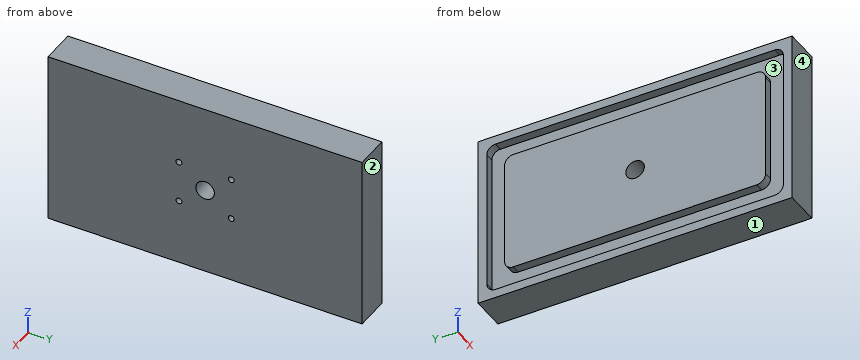
Autodesk Inventor part; units mm, degrees
ref_plane "YZ Plane" through (0, 0, 0) normal (1, 0, 0) x (0, 1, 0)
ref_plane "XZ Plane" through (0, 0, 0) normal (0, 1, 0) x (-1, 0, 0)
ref_plane "XY Plane" through (0, 0, 0) normal (0, 0, 1) x (1, 0, 0)
sketch "Sketch1" plane through (0, 0, 0) normal (1, 0, 0) x (0, 1, 0)
  line L0 (57.15, 31.75) -> (-57.15, 31.75)
  line L1 (-57.15, 31.75) -> (-57.15, -31.75)
  line L2 (-57.15, -31.75) -> (57.15, -31.75)
  line L3 (57.15, -31.75) -> (57.15, 31.75)
  line L4 (-50.8, 25.4) -> (50.8, 25.4)
  line L5 (50.8, 25.4) -> (50.8, -25.4)
  line L6 (50.8, -25.4) -> (-50.8, -25.4)
  line L7 (-50.8, -25.4) -> (-50.8, 25.4)
  point P0 (0, 0)
  point P1 (0, -31.75)
  point P2 (57.15, 0)
  point P3 (0, 25.4)
  point P4 (-50.8, 0)
  dimension "d0" = 63.5
  dimension "d1" = 114.3
  dimension "d14" = 50.8
  dimension "d15" = 101.6
extrude "Extrusion1" add sketch "Sketch1" along normal blind 12.7 contours L3 L2 L1 L0 | L4 L5 L6 L7
sketch "Sketch2" plane through (12.7, 0, 0) normal (1, 0, 0) x (0, 0, -1)
  line L0 (-7.62, -9.525) -> (7.62, 9.525) construction
  line L1 (-7.62, 9.525) -> (7.62, -9.525) construction
  circle A0 centre (0, 0) radius 3.3734
  dimension "d5" = 19.05
  dimension "d12" = 6.7469
  dimension "d13" = 15.24
sketch "Sketch3" plane through (0, 0, 0) normal (-1, 0, 0) x (0, 0, 1)
  line L0 (-28.575, -53.975) -> (28.575, -53.975)
  line L1 (28.575, -53.975) -> (28.575, 53.975)
  line L2 (28.575, 53.975) -> (-28.575, 53.975)
  line L3 (-28.575, 53.975) -> (-28.575, -53.975)
  line L4 (22.098, 47.498) -> (22.098, -47.498)
  line L5 (22.098, -47.498) -> (-22.098, -47.498)
  line L6 (-22.098, -47.498) -> (-22.098, 47.498)
  line L7 (-22.098, 47.498) -> (22.098, 47.498)
  point P0 (0, 0)
  point P1 (0, -53.975)
  point P2 (-28.575, 0)
  point P3 (0, 0)
  point P4 (28.575, 0)
  point P5 (0, 53.975)
  dimension "d16" = 107.95
  dimension "d17" = 57.15
  dimension "d31" = 6.477
extrude "Extrusion3" cut sketch "Sketch3" against normal blind 3.175
extrude "Extrusion4" cut sketch "Sketch2" against normal through all
hole "Hole1" at (12.7, -9.525, 7.62) at (12.7, 9.525, 7.62) at (12.7, 9.525, -7.62) at (12.7, -9.525, -7.62) direction (-1, 0, 0) diameter 2.159 depth 8.8646 tip angle 118
fillet "Fillet1" radius 3.175 8 edges at (1.5875, 53.975, 28.575) (1.5875, -47.498, 22.098) (1.5875, -47.498, -22.098) (1.5875, -53.975, -28.575) (1.5875, 47.498, -22.098) (1.5875, -53.975, 28.575) (1.5875, 53.975, -28.575) (1.5875, 47.498, 22.098)
properties part number "plate" material "Aluminum 6061"
Read the model definition and answer for the solid it produces. Units are mm, in the model's axes. Face numbers are marked on the shaded views. Give positions to 0.01 mm unless a question says otherwise; leave off trailing zeros. Write each loop counter-clockwise with the first axis right and the second up, starting at its lowest first coordinate (ties: lowest second). Pieces come first, ordered by that corner, then holes. Notation, with made-up numbers: (87.25, 14) -> (134.25, 14) arc R21 ccw to (134.25, 18) -> close; hole circle Ø11 at (43, 61.5). An arc over 180 degrees is marked (long way). Answer in a Markdown table with one row per item.
1) This flat-tipped pin is pushed along its axis until it touches: pin 1 Ø9 at (y, z) = (0, 0) entering from -X. Where does it stop, or does it pass through?
Results list:
| item | result |
|---|---|
| pin 1 | x = 0 |
2) Section C-C on y = 0 is taken. Give the vertices of the cut face in (x, z) (3 decimals).
Results list:
| item | result |
|---|---|
| outline | (0, -31.75) -> (12.7, -31.75) -> (12.7, -3.373) -> (0, -3.373) -> (0, -22.098) -> (3.175, -22.098) -> (3.175, -28.575) -> (0, -28.575) -> close; (0, 3.373) -> (12.7, 3.373) -> (12.7, 31.75) -> (0, 31.75) -> (0, 28.575) -> (3.175, 28.575) -> (3.175, 22.098) -> (0, 22.098) -> close |
3) Section A-A on x = 1.5 is taken. Give the vertices of the cut face in (y, z) (3 decimals).
Results list:
| item | result |
|---|---|
| outline | (-57.15, -31.75) -> (57.15, -31.75) -> (57.15, 31.75) -> (-57.15, 31.75) -> close; (-47.498, -18.923) arc R3.175 ccw to (-44.323, -22.098) -> (44.323, -22.098) arc R3.175 ccw to (47.498, -18.923) -> (47.498, 18.923) arc R3.175 ccw to (44.323, 22.098) -> (-44.323, 22.098) arc R3.175 ccw to (-47.498, 18.923) -> close; hole (-53.975, -25.4) arc R3.175 ccw to (-50.8, -28.575) -> (50.8, -28.575) arc R3.175 ccw to (53.975, -25.4) -> (53.975, 25.4) arc R3.175 ccw to (50.8, 28.575) -> (-50.8, 28.575) arc R3.175 ccw to (-53.975, 25.4) -> close; hole circle Ø6.747 at (0, 0) |
4) Section D-D on z = 10 is taken. Give the vertices of the cut face in (x, y) (3 decimals), plus the area to 3 significant figures.
Results list:
| item | result |
|---|---|
| outline | (0, -57.15) -> (12.7, -57.15) -> (12.7, 57.15) -> (0, 57.15) -> (0, 53.975) -> (3.175, 53.975) -> (3.175, 47.498) -> (0, 47.498) -> (0, -47.498) -> (3.175, -47.498) -> (3.175, -53.975) -> (0, -53.975) -> close |
| area | 1,410 mm^2 |
5) Determine the mould class of the marked faces 1, 2, 3 and 4 for opening direction Y: released by +Y, released by -Y, zero draft, split by the parting line, or undercut.
Results list:
| item | result |
|---|---|
| face 1 | zero draft |
| face 2 | released by +Y |
| face 3 | undercut |
| face 4 | released by -Y |
6) Section B-B on z = 0 is taken. Give the vertices of the cut face in (x, y) (3 decimals), plus the area to 3 significant figures.
Results list:
| item | result |
|---|---|
| outline | (0, -57.15) -> (12.7, -57.15) -> (12.7, -3.373) -> (0, -3.373) -> (0, -47.498) -> (3.175, -47.498) -> (3.175, -53.975) -> (0, -53.975) -> close; (0, 3.373) -> (12.7, 3.373) -> (12.7, 57.15) -> (0, 57.15) -> (0, 53.975) -> (3.175, 53.975) -> (3.175, 47.498) -> (0, 47.498) -> close |
| area | 1,320 mm^2 |
7) Straight lines are drawn through the part: line 1 (Y direction, x = 7, z = -7.62); line 2 (Y direction, x = 1, z = -15) (3 decimals); line 3 (Z direction, x = 3.75, y = -10). For each, find the intervals that lie inside material, in ascending order. Write a range as [from, to].
Results list:
| item | result |
|---|---|
| line 1 | [-57.15, -10.6], [-8.45, 8.45], [10.6, 57.15] |
| line 2 | [-57.15, -53.975], [-47.498, 47.498], [53.975, 57.15] |
| line 3 | [-31.75, -8.43], [-6.81, 6.81], [8.43, 31.75] |
